Read the model definition and answer for the solid it produces. Units are mm, in the model's axes. Face numbers are marked on the shaded views. A direction names the side the tool comes from. Coordinates: 2 decimals unless noted, no trailing zeros. Loops run counter-clockwise (first coordinate to the right, second up) from the corner with the lowest first, then second, coordinate; pieces in that order, holes last. Notation, with made-up numbers: (68.5, 22.25) -> (120.5, 22.25) arc R14 cw to (120.5, 29.25) -> close; hole circle Ø3 at (19, -2.75). An arc over 180 degrees is marked (long way). One line per question, with ' | ' between items. Start each with the question number.
```python
from build123d import *

# Parameters (mm, degrees)
SKETCH1_W           = 127
SKETCH1_H           = 38.1
BOSS_EXTRUDE1_DEPTH = 3.175
SKETCH3_R           = 12.7
BOSS_EXTRUDE2_DEPTH = 38.1
SKETCH4_R           = 6.35
CUT_EXTRUDE1_DEPTH  = 76.134213245


with BuildPart() as part:
    # Sketch1 → Boss-Extrude1 (new, symmetric)
    with BuildSketch(Plane(origin=(0, 0, 0), x_dir=(1, 0, 0), z_dir=(0, 1, 0))):
        Rectangle(SKETCH1_W, SKETCH1_H)
    extrude(amount=BOSS_EXTRUDE1_DEPTH, both=True)

    # Sketch3 → Boss-Extrude2 (add)
    with BuildSketch(Plane.XY.offset(19.05)):
        Circle(SKETCH3_R)
    extrude(amount=-BOSS_EXTRUDE2_DEPTH)

    # Sketch4 → Cut-Extrude1 (cut, through all)
    with BuildSketch(Plane.XY.offset(19.05)):
        Circle(SKETCH4_R)
    extrude(amount=-CUT_EXTRUDE1_DEPTH, mode=Mode.SUBTRACT)


solid = part.part
```
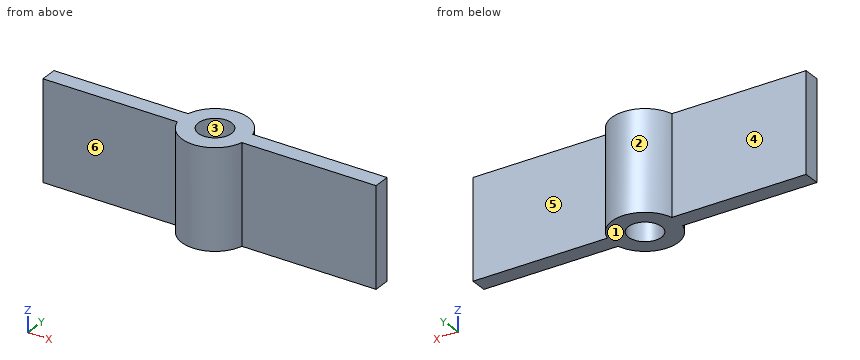
(1) Find the intervals of material crossed by probe 1 along Y at (x, z) = (0, 10.5); probe 2 along Y at (x, z) = (38, 17.5) (3 decimals); probe 3 along X at (y, z) = (-4.25, -8), in increasing order. Write a range as from..to.
(2) Section C-C on z = 14.5 is taken. Write down the section's boundary in (x, y) (3 decimals).
(3) Each of these flat-tipped pins is pushed along its axis until it touches: pin 1 Ø11.5 at (x, z) = (-30.5, 8) entering from +Y (3 decimals); pin 2 Ø1.5 at (y, z) = (5.5, -0.5) entering from -X; pin 3 Ø3 at (x, z) = (2, -5.5) entering from -Y; pin 4 Ø1 at (x, y) = (13, 7) entering from -Z. Where does it stop, or does it pass through?
(4) Determine the mould class of the marked faces 1, 2 and 3 for opening direction X: +X half, -X half, draft (parallel to the pull), parting line (faces both ways), or undercut.
(5) Section B-B on y = 0 is taken. Write down the section's boundary in (x, z), plus the area to 3 significant figures.
(6) A tool of negligible diameter and unlimited length cuts with its end or side. For the marked faces 4, 5 and 6, from which of +Z, -Z, +X, -X, +Y, -Y can it reach the whole face along a straight path? Write none if from no direction.
(7) Section A-A on x = 0 is taken. Write down the section's boundary in (y, z), plus the area to 3 significant figures.
(8) Section D-D on x = -15 is taken. Write down the section's boundary in (y, z) (3 decimals), plus the area to 3 significant figures.
Working result:
1) probe 1: y = -12.7..-6.35, 6.35..12.7 | probe 2: y = -3.175..3.175 | probe 3: x = -11.97..-4.72, 4.72..11.97
2) outline: (-63.5, -3.175) -> (-12.297, -3.175) arc R12.7 ccw to (12.297, -3.175) -> (63.5, -3.175) -> (63.5, 3.175) -> (12.297, 3.175) arc R12.7 ccw to (-12.297, 3.175) -> (-63.5, 3.175) -> close; hole circle Ø12.7 at (0, 0)
3) pin 1: stops at y = 3.175 | pin 2: stops at x = -11.78 | pin 3: stops at y = -12.69 | pin 4: passes through
4) face 1: draft | face 2: parting line | face 3: undercut
5) outline: (-63.5, -19.05) -> (-6.35, -19.05) -> (-6.35, 19.05) -> (-63.5, 19.05) -> close; (6.35, -19.05) -> (63.5, -19.05) -> (63.5, 19.05) -> (6.35, 19.05) -> close | area: 4,350 mm2
6) face 4: +Z, -Z, -X, +Y | face 5: +Z, -Z, +X, +Y | face 6: +Z, -Z, -X, -Y
7) outline: (-12.7, -19.05) -> (-6.35, -19.05) -> (-6.35, 19.05) -> (-12.7, 19.05) -> close; (6.35, -19.05) -> (12.7, -19.05) -> (12.7, 19.05) -> (6.35, 19.05) -> close | area: 484 mm2
8) outline: (-3.175, -19.05) -> (3.175, -19.05) -> (3.175, 19.05) -> (-3.175, 19.05) -> close | area: 242 mm2
